The model under review builds one solid part; all positions refer to its coordinate system, in mm. Round coordinates to 2 decimals unless told otherwise and drop trailing zeros. One line per item, written item: value. Start each with the question number.
from build123d import *

# Parameters (mm, degrees)
F0_W     = 200
F0_H     = 145
F0_W_2   = 10
F0_H_2   = 3
F0_R     = 1.5
F0_W_3   = 3
F0_H_3   = 10
F0_R_2   = 3.25
F0_H_4   = 135
F0_W_4   = 41
F0_H_5   = 20.5
F1_DEPTH = 3


with BuildPart() as f1:
    # F0 (on Top) → F1 (new body)
    with BuildSketch(Plane.XY):
        with Locations((212.266122, 82.063026)):
            Rectangle(F0_W, F0_H)
        with Locations((153.266122, 14.563026)):
            Rectangle(F0_W_2, F0_H_2, mode=Mode.SUBTRACT)
        with Locations((164.766122, 14.563026)):
            Circle(F0_R, mode=Mode.SUBTRACT)
        with Locations((176.266122, 14.563026)):
            Rectangle(F0_W_2, F0_H_2, mode=Mode.SUBTRACT)
        with Locations((117.264537, 70.563026)):
            Rectangle(F0_W_3, F0_H_3, mode=Mode.SUBTRACT)
        with Locations((124.266122, 77.063026)):
            Circle(F0_R, mode=Mode.SUBTRACT)
        with Locations((171.266122, 77.063026)):
            Circle(F0_R, mode=Mode.SUBTRACT)
        with Locations((248.266122, 14.563026)):
            Rectangle(F0_W_2, F0_H_2, mode=Mode.SUBTRACT)
        with Locations((259.766122, 14.563026)):
            Circle(F0_R, mode=Mode.SUBTRACT)
        with Locations((260.766122, 22.063026)):
            Circle(F0_R_2, mode=Mode.SUBTRACT)
        with Locations((271.266122, 14.563026)):
            Rectangle(F0_W_2, F0_H_2, mode=Mode.SUBTRACT)
        with Locations((299.266122, 22.063026)):
            Circle(F0_R_2, mode=Mode.SUBTRACT)
        with Locations((260.766122, 60.563026)):
            Circle(F0_R_2, mode=Mode.SUBTRACT)
        with Locations((238.266122, 79.563026)):
            Rectangle(F0_W_2, F0_H_2, mode=Mode.SUBTRACT)
        with Locations((249.766122, 79.563026)):
            Circle(F0_R, mode=Mode.SUBTRACT)
        with Locations((261.266122, 79.563026)):
            Rectangle(F0_W_2, F0_H_2, mode=Mode.SUBTRACT)
        with Locations((299.266122, 60.563026)):
            Circle(F0_R_2, mode=Mode.SUBTRACT)
        with Locations((307.266122, 82.063026)):
            Rectangle(F0_W_3, F0_H_4, mode=Mode.SUBTRACT)
        with Locations((117.266122, 82.063026)):
            Circle(F0_R, mode=Mode.SUBTRACT)
        with Locations((124.266122, 87.063026)):
            Circle(F0_R, mode=Mode.SUBTRACT)
        with Locations((117.264537, 93.563026)):
            Rectangle(F0_W_3, F0_H_3, mode=Mode.SUBTRACT)
        with Locations((147.766122, 82.063026)):
            Rectangle(F0_W_4, F0_H_5, mode=Mode.SUBTRACT)
        with Locations((171.266122, 87.063026)):
            Circle(F0_R, mode=Mode.SUBTRACT)
        with Locations((192.264537, 103.063026)):
            Rectangle(F0_W_3, F0_H_3, mode=Mode.SUBTRACT)
        with Locations((192.266122, 114.563026)):
            Circle(F0_R, mode=Mode.SUBTRACT)
        with Locations((153.266122, 149.563026)):
            Rectangle(F0_W_2, F0_H_2, mode=Mode.SUBTRACT)
        with Locations((192.264537, 126.063026)):
            Rectangle(F0_W_3, F0_H_3, mode=Mode.SUBTRACT)
        with Locations((164.766122, 149.563026)):
            Circle(F0_R, mode=Mode.SUBTRACT)
        with Locations((176.266122, 149.563026)):
            Rectangle(F0_W_2, F0_H_2, mode=Mode.SUBTRACT)
        with Locations((260.766122, 103.563026)):
            Circle(F0_R_2, mode=Mode.SUBTRACT)
        with Locations((299.266122, 103.563026)):
            Circle(F0_R_2, mode=Mode.SUBTRACT)
        with Locations((260.766122, 142.063026)):
            Circle(F0_R_2, mode=Mode.SUBTRACT)
        with Locations((248.266122, 149.563026)):
            Rectangle(F0_W_2, F0_H_2, mode=Mode.SUBTRACT)
        with Locations((259.766122, 149.563026)):
            Circle(F0_R, mode=Mode.SUBTRACT)
        with Locations((271.266122, 149.563026)):
            Rectangle(F0_W_2, F0_H_2, mode=Mode.SUBTRACT)
        with Locations((299.266122, 142.063026)):
            Circle(F0_R_2, mode=Mode.SUBTRACT)
    extrude(amount=F1_DEPTH)


solid = f1.part
Item 1: Consider section A-A, the plane z = 1.15. Count the separate pieces of the cut face and the enclosed holes in it, then the cut area to 3 significant figures.
Item 2: The part is to be moulded in two halves that separate along X. For faces 1 (the cylindrical face through (302.366, 61.539, 1.479)), 2 (the flat face through (211, 83, 3)), 3 (the cylindrical face through (263.866, 61.539, 1.479)), say which applies: pulls with the +X half, pulls with the -X half, needs draft (parallel to the pull), parting line crosses it, or undercut.
Item 3: Wall thickness on L1, parallel to X at y = 68.5, z = 2.5; L2, parallel to Y at x = 252, z = 2.3; L3, parallel to Y at x = 124.5, z = 1.5: over which ranges is each line inside the solid? List them lowest first.
Computed:
1. separate pieces: 1
1. enclosed holes: 35
1. area: 27,000 mm^2
2. face 1: undercut
2. face 2: needs draft
2. face 3: undercut
3. L1: x = 112.27 to 115.76, 118.76 to 305.77, 308.77 to 312.27
3. L2: y = 9.56 to 13.06, 16.06 to 148.06, 151.06 to 154.56
3. L3: y = 9.56 to 75.58, 78.54 to 85.58, 88.54 to 154.56
